```python
from build123d import *

# Parameters (mm, degrees)
F0_W     = 30
F0_H     = 30
F1_DEPTH = 1.6
F2_W     = 13
F2_H     = 9.4
F3_DEPTH = 25
F2_W_2   = 17
F2_H_2   = 13.4
F4_DEPTH = 15
F5_DEPTH = 25


with BuildPart() as f1:
    # F0 (on Top) → F1 (new body)
    with BuildSketch(Plane.XY):
        with Locations((15, -15)):
            Rectangle(F0_W, F0_H)
    extrude(amount=F1_DEPTH)

    # F2 (on face) → F3 (cut)
    with BuildSketch(Plane.XY.offset(1.6)):
        with Locations((15, -7.5)):
            Rectangle(F2_W, F2_H)
    extrude(amount=-F3_DEPTH, mode=Mode.SUBTRACT)

    # F2 (on face) → F4 (join)
    with BuildSketch(Plane.XY.offset(1.6)):
        with Locations((15, -22.5)):
            Rectangle(F2_W_2, F2_H_2)
        with Locations((15, -22.5)):
            Rectangle(F2_W, F2_H, mode=Mode.SUBTRACT)
    extrude(amount=F4_DEPTH)

    # F2 (on face) → F5 (cut)
    with BuildSketch(Plane.XY.offset(1.6)):
        with Locations((15, -22.5)):
            Rectangle(F2_W, F2_H)
    extrude(amount=-F5_DEPTH, mode=Mode.SUBTRACT)


solid = f1.part
```
CAD build for the part. Positions are in the model's coordinates, mm. A direction names the side the tool comes from. Coordinates: 2 decimals unless noted, no trailing zeros. Order: outer loops, then holes, each group sorted by start corner. A loop starts at its lowest first (then second) coordinate and runs counter-clockwise, first axis right, second up. Notation, with made-up numbers: M -36,11 L -16,11 A24 cw -16,44 Z; hole C 86,-30 d11. An arc over 180 degrees is marked long. Write each question's results on one line, items separated by ' | '. Start each with the question number.
Q1. Cut at B-B (y = -8.25). List the corners of the cut face in (x, z).
Q2. Cut at A-A (x = 9.75). List the corners of the cut face in (y, z), then the cut area to 3 significant figures.
Q3. Which spindle directions (+Z, -Z, +X, -X, +Y, -Y) get a long thin tool onto all of the face, cutting with end or side? Do faces 4 (the flat face through (8.5, -23, 8)), 5 (the flat face through (6.5, -23, 9)), 6 (the flat face through (15, -15.8, 9)), 7 (the flat face through (15, -29.2, 9)). Say none if no direction does.
Q4. Drill centre lines: probe 1 along Y at (x, z) = (15, 3.25); probe 2 along X at (y, z) = (-25.5, 5.25); probe 3 along Z at (x, y) = (1.5, -23.75). Where is each one in solid material? Low to high. Write a range as from..to.
Q5. Cut at C-C (z = 8.25). List the corners of the cut face in (x, y).
Q6. Pull direction Y, two halves, no side cores. Call faces 1 (the flat face through (15, -12.2, 1)), 2 (the flat face through (15, -30, 1)), 3 (the flat face through (23.5, -23, 9)): +Y half, -Y half, draft (parallel to the pull), parting line (faces both ways), or undercut.
Q7. Flat gauge pins, fed straight in: P1, Ø5, axis at x = 4.5, z = 15, coming from the +Y side; P2, Ø4, axis at y = -24, z = 10, coming from the +X side; P3, Ø9, axis at x = 22, y = -10, coming from the +Z side. Where does each tip first touch, or does it go through?
Q8. Cut at D-D (y = -17.25). List the corners of the cut face in (x, z).
Found:
1) outline: M 0,0 L 8.5,0 L 8.5,1.6 L 0,1.6 Z; M 21.5,0 L 30,0 L 30,1.6 L 21.5,1.6 Z
2) outline: M -30,0 L -27.2,0 L -27.2,16.6 L -29.2,16.6 L -29.2,1.6 L -30,1.6 Z; M -17.8,0 L -12.2,0 L -12.2,1.6 L -15.8,1.6 L -15.8,16.6 L -17.8,16.6 Z; M -2.8,0 L 0,0 L 0,1.6 L -2.8,1.6 Z | area: 77.9 mm²
3) face 4: +Z, -Z | face 5: +Z, -X, +Y, -Y | face 6: +Z, +X, -X, +Y | face 7: +Z, +X, -X, -Y
4) probe 1: -29.2..-27.2, -17.8..-15.8 | probe 2: 6.5..8.5, 21.5..23.5 | probe 3: 0..1.6
5) outline: M 6.5,-29.2 L 23.5,-29.2 L 23.5,-15.8 L 6.5,-15.8 Z; hole M 8.5,-27.2 L 21.5,-27.2 L 21.5,-17.8 L 8.5,-17.8 Z
6) face 1: undercut | face 2: -Y half | face 3: draft
7) P1: y = -15.8 | P2: x = 23.5 | P3: z = 1.6
8) outline: M 0,0 L 30,0 L 30,1.6 L 23.5,1.6 L 23.5,16.6 L 6.5,16.6 L 6.5,1.6 L 0,1.6 Z
